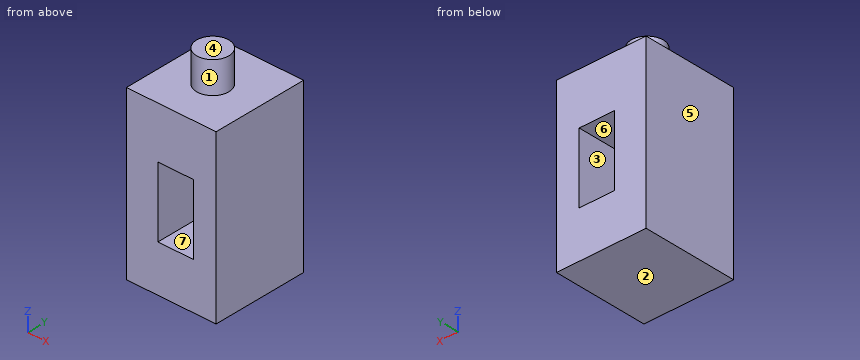
```python
from build123d import *

# Parameters (mm, degrees)
F0_W     = 77.007651329
F0_H     = 135.7397735119
F1_DEPTH = 72.2800772637
F2_R     = 12.98884786
F3_DEPTH = 25.4
F4_W     = 22.6057656109
F4_H     = 36.8559285998
F5_DEPTH = 49.8851463199
F6_W     = 28.5666175187
F6_H     = 56.4576983452
F7_DEPTH = 77.007651329


with BuildPart() as f1:
    # F0 (on Right) → F1 (new body)
    with BuildSketch(Plane.YZ):
        with Locations((-24.8167514801, 61.0263496637)):
            Rectangle(F0_W, F0_H)
    extrude(amount=F1_DEPTH)

    # F2 (on face) → F3 (join)
    with BuildSketch(Plane.XY.offset(128.8962364197)):
        with Locations((35.1639688015, -25.7027596235)):
            Circle(F2_R)
    extrude(amount=F3_DEPTH)

    # F4 (on face) → F5 (cut)
    with BuildSketch(Plane.YZ.offset(72.2800772637)):
        with Locations((-26.0762441903, 56.855943054)):
            Rectangle(F4_W, F4_H)
    extrude(amount=F5_DEPTH, mode=Mode.SUBTRACT)

    # F6 (on face) → F7 (cut, through all)
    with BuildSketch(Plane.XZ.offset(63.3205771446)):
        with Locations((39.6464411169, 59.0323209763)):
            Rectangle(F6_W, F6_H)
    extrude(amount=-F7_DEPTH, mode=Mode.SUBTRACT)


solid = f1.part
```
Build history of the part. All positions in model axes, mm. Face numbers are marked on the shaded views. A direction names the side the tool comes from. Coordinates: 2 decimals unless noted, no trailing zeros. Write each loop counter-clockwise with the first axis right and the second up, starting at its lowest first coordinate (ties: lowest second). Pieces come first, ordered by that corner, then holes.
1. Band-saw the part on B-B, the plane y = -3.5. Give the cut face in (x, z).
Answer block:
outline: (0, -6.84) - (72.28, -6.84) - (72.28, 128.9) - (0, 128.9) - close; hole (25.36, 30.8) - (53.93, 30.8) - (53.93, 87.26) - (25.36, 87.26) - close
2. Band-saw the part on D-D, the plane x = 60. Give the cut face in (y, z), and give its area (3 significant figures).
Answer block:
outline: (-63.32, -6.84) - (13.69, -6.84) - (13.69, 128.9) - (-63.32, 128.9) - close
area: 10,500 mm2
3. Drop flat-ended pins along their axis: pin 1 (6 mm diameter, centred on y = -50.5, z = 68, fed in from -X); pin 2 (3 mm diameter, centred on x = 62.5, y = -48, fed in from +Z). Give the stop position or say it passes through.
Answer block:
pin 1: stops at x = 0
pin 2: stops at z = 128.9
4. Drill centre lines: probe 1 along X at (y, z) = (-38.5, 55.5); probe 2 along Z at (x, y) = (34.5, 6); probe 3 along Z at (x, y) = (58.5, -37). Where is each one in solid material? Low to high.
Answer block:
probe 1: x = 0 to 25.36, 53.93 to 72.28
probe 2: z = -6.84 to 30.8, 87.26 to 128.9
probe 3: z = -6.84 to 128.9
5. Pull direction X, two halves, no side cores. Call the marked faces 4, 5, 6 and 7: released by +X, released by -X, zero draft, split by the parting line, or undercut.
Answer block:
face 4: zero draft
face 5: released by -X
face 6: undercut
face 7: undercut
6. Band-saw the part on A-A, the plane z = 63. Give the cut face in (x, y).
Answer block:
outline: (0, -63.32) - (25.36, -63.32) - (25.36, 13.69) - (0, 13.69) - close; (53.93, -63.32) - (72.28, -63.32) - (72.28, 13.69) - (53.93, 13.69) - close
7. Band-saw the part on C-C, the plane x = 39.5. Give the cut face in (y, z), and give its area (3 significant figures).
Answer block:
outline: (-63.32, -6.84) - (13.69, -6.84) - (13.69, 30.8) - (-63.32, 30.8) - close; (-63.32, 87.26) - (13.69, 87.26) - (13.69, 128.9) - (-13.46, 128.9) - (-13.46, 154.3) - (-37.95, 154.3) - (-37.95, 128.9) - (-63.32, 128.9) - close
area: 6,730 mm2
8. 3-axis set-ups, long thin cutter, end or side, ignore diameter. For the marked faces 1, 2 and 3: which of +Z, -Z, +X, -X, +Y, -Y reach the whole face in a straight line?
Answer block:
face 1: +Z
face 2: -Z, +X, -X, +Y, -Y
face 3: +Y, -Y
